Read the model definition and answer for the solid it produces. Units are mm, in the model's axes. Coordinates: 2 decimals unless noted, no trailing zeros. Write each loop counter-clockwise with the first axis right and the second up, starting at its lowest first coordinate (ties: lowest second). Pieces come first, ordered by that corner, then holes. Notation, with made-up numbers: (-39.75, 57) -> (-34.75, 57) arc R37 ccw to (-34.75, 93) -> close; hole circle Ø9 at (23.25, 26.25). An arc over 180 degrees is marked (long way). Answer in a Markdown table with one row per item. Add a question column.
Item 1: Straight lines are drawn through the part: line 1 (Z direction, x = 19.5, y = -0.2); line 2 (X direction, y = 1.35, z = -0.7). For each, find the intervals that lie inside material, in ascending order. Write a range as from..to.
Item 2: Section A-A on x = -17 is taken. Write down the section's boundary in (y, z), then the cut area to 3 significant figures.
Item 3: Given pin 1 Ø1 at (x, z) = (-31, 1.5) entering from -Y, flat-ended and moving along its own axis, determine where the tip first touches the part or whether it passes through.
Solid Edge part; units mm, degrees
sketch "Sketch1" plane through (0, 0, 0) normal (1, 0, 0) x (0, 1, 0)
  circle A0 centre (0, 0) radius 2
extrude "Protrusion1" add sketch "Sketch1" along normal mid plane 105
cosmetic_thread "Thread_1" thread depth 8
cosmetic_thread "Thread_2" thread depth 8
chamfer "Chamfer_1" distance 0.5 angle 45 1 edges at (52.5, -2, 0) measured on face at (52.5, 1.2933, -1.3733)
chamfer "Chamfer_2" distance 0.5 angle 45 1 edges at (-52.5, -2, 0) measured on face at (-52.5, 1.2933, -1.3733)
Results below:
| question | item | result |
|---|---|---|
| 1 | line 1 | z = -1.99..1.99 |
| 1 | line 2 | x = -52.48..52.48 |
| 2 | outline | circle Ø4 at (0, 0) |
| 2 | area | 12.6 mm2 |
| 3 | pin 1 | stops at y = -1.73 |
